```python
from build123d import *

# Parameters (mm, degrees)
SKETCH_1_R          = 18
SKETCH_1_R_2        = 1.6
SKETCH_1_R_3        = 2.6
SKETCH_1_R_4        = 1.35
EXTRUDE_1_DEPTH     = 3
CUT_EXTRUDE_1_REACH = 132.882
SKETCH_2_R          = 24


with BuildPart() as part:
    # 草图1 → 凸台-拉伸1 (new body)
    with BuildSketch(Plane(origin=(0, 0, 0), x_dir=(1, 0, 0), z_dir=(0, 1, 0))):
        with BuildLine():
            Line((100, -47.5), (-100, -47.5))
            ThreePointArc((-100, -47.5), (-121.921951267, 0), (-100, 47.5))
            Line((-100, 47.5), (100, 47.5))
            ThreePointArc((100, 47.5), (121.921951267, 0), (100, -47.5))
        make_face()
        with Locations(Location((77.5, 0, 0), (0, 0, 270))):
            Circle(SKETCH_1_R, mode=Mode.SUBTRACT)
        with Locations(Location((77.5, 37, 0), (0, 0, 270))):
            Circle(SKETCH_1_R_2, mode=Mode.SUBTRACT)
        with Locations(Location((103.662950904, 26.162950904, 0), (0, 0, 270))):
            Circle(SKETCH_1_R_2, mode=Mode.SUBTRACT)
        with Locations(Location((114.5, 0, 0), (0, 0, 270))):
            Circle(SKETCH_1_R_2, mode=Mode.SUBTRACT)
        with Locations(Location((103.662950904, -26.162950904, 0), (0, 0, 270))):
            Circle(SKETCH_1_R_2, mode=Mode.SUBTRACT)
        with Locations(Location((77.5, -37, 0), (0, 0, 270))):
            Circle(SKETCH_1_R_2, mode=Mode.SUBTRACT)
        with Locations(Location((51.337049096, -26.162950904, 0), (0, 0, 270))):
            Circle(SKETCH_1_R_2, mode=Mode.SUBTRACT)
        with Locations(Location((40.5, 0, 0), (0, 0, 270))):
            Circle(SKETCH_1_R_2, mode=Mode.SUBTRACT)
        with Locations(Location((51.337049096, 26.162950904, 0), (0, 0, 270))):
            Circle(SKETCH_1_R_2, mode=Mode.SUBTRACT)
        with Locations(Location((-51.337049096, 26.162950904, 0), (0, 0, 270))):
            Circle(SKETCH_1_R_2, mode=Mode.SUBTRACT)
        with Locations(Location((-40.5, 0, 0), (0, 0, 270))):
            Circle(SKETCH_1_R_2, mode=Mode.SUBTRACT)
        with Locations(Location((-51.337049096, -26.162950904, 0), (0, 0, 270))):
            Circle(SKETCH_1_R_2, mode=Mode.SUBTRACT)
        with Locations(Location((-77.5, -37, 0), (0, 0, 270))):
            Circle(SKETCH_1_R_2, mode=Mode.SUBTRACT)
        with Locations(Location((-103.662950904, -26.162950904, 0), (0, 0, 270))):
            Circle(SKETCH_1_R_2, mode=Mode.SUBTRACT)
        with Locations(Location((-114.5, 0, 0), (0, 0, 270))):
            Circle(SKETCH_1_R_2, mode=Mode.SUBTRACT)
        with Locations(Location((-103.662950904, 26.162950904, 0), (0, 0, 270))):
            Circle(SKETCH_1_R_2, mode=Mode.SUBTRACT)
        with Locations(Location((-77.5, 37, 0), (0, 0, 270))):
            Circle(SKETCH_1_R_2, mode=Mode.SUBTRACT)
        with Locations(Location((-77.5, 0, 0), (0, 0, 270))):
            Circle(SKETCH_1_R, mode=Mode.SUBTRACT)
        with Locations(Location((-10, -30.5, 0), (0, 0, 270))):
            Circle(SKETCH_1_R_3, mode=Mode.SUBTRACT)
        with Locations(Location((10, -30.5, 0), (0, 0, 270))):
            Circle(SKETCH_1_R_3, mode=Mode.SUBTRACT)
        with Locations(Location((-40, -30.5, 0), (0, 0, 270))):
            Circle(SKETCH_1_R_3, mode=Mode.SUBTRACT)
        with Locations(Location((40, -30.5, 0), (0, 0, 270))):
            Circle(SKETCH_1_R_3, mode=Mode.SUBTRACT)
        with Locations(Location((40, 30.5, 0), (0, 0, 270))):
            Circle(SKETCH_1_R_3, mode=Mode.SUBTRACT)
        with Locations(Location((10, 30.5, 0), (0, 0, 270))):
            Circle(SKETCH_1_R_3, mode=Mode.SUBTRACT)
        with Locations(Location((-10, 30.5, 0), (0, 0, 270))):
            Circle(SKETCH_1_R_3, mode=Mode.SUBTRACT)
        with Locations(Location((-40, 30.5, 0), (0, 0, 270))):
            Circle(SKETCH_1_R_3, mode=Mode.SUBTRACT)
        with Locations(Location((-30, -40.5, 0), (0, 0, 270))):
            Circle(SKETCH_1_R_2, mode=Mode.SUBTRACT)
        with Locations(Location((-40, -40.5, 0), (0, 0, 270))):
            Circle(SKETCH_1_R_2, mode=Mode.SUBTRACT)
        with Locations(Location((40, -40.5, 0), (0, 0, 270))):
            Circle(SKETCH_1_R_2, mode=Mode.SUBTRACT)
        with Locations(Location((30, -40.5, 0), (0, 0, 270))):
            Circle(SKETCH_1_R_2, mode=Mode.SUBTRACT)
        with Locations(Location((-40, 41, 0), (0, 0, 270))):
            Circle(SKETCH_1_R_2, mode=Mode.SUBTRACT)
        with Locations(Location((-30, 41, 0), (0, 0, 270))):
            Circle(SKETCH_1_R_2, mode=Mode.SUBTRACT)
        with Locations(Location((30, 41, 0), (0, 0, 270))):
            Circle(SKETCH_1_R_2, mode=Mode.SUBTRACT)
        with Locations(Location((40, 41, 0), (0, 0, 270))):
            Circle(SKETCH_1_R_2, mode=Mode.SUBTRACT)
        with Locations(Location((100, 37.5, 0), (0, 0, 270))):
            Circle(SKETCH_1_R_2, mode=Mode.SUBTRACT)
        with Locations(Location((100, -37.5, 0), (0, 0, 270))):
            Circle(SKETCH_1_R_2, mode=Mode.SUBTRACT)
        with Locations(Location((-100, -37.5, 0), (0, 0, 270))):
            Circle(SKETCH_1_R_2, mode=Mode.SUBTRACT)
        with Locations(Location((-100, 37.5, 0), (0, 0, 270))):
            Circle(SKETCH_1_R_2, mode=Mode.SUBTRACT)
        with Locations(Location((-30.5, 8, 0), (0, 0, 270))):
            Circle(SKETCH_1_R_4, mode=Mode.SUBTRACT)
        with BuildLine():
            Line((-36, 20), (-25, 20))
            ThreePointArc((-25, 20), (-23.585786438, 19.414213562), (-23, 18))
            Line((-23, 18), (-23, 12))
            ThreePointArc((-23, 12), (-23.585786438, 10.585786438), (-25, 10))
            Line((-25, 10), (-36, 10))
            ThreePointArc((-36, 10), (-37.414213562, 10.585786438), (-38, 12))
            Line((-38, 12), (-38, 18))
            ThreePointArc((-38, 18), (-37.414213562, 19.414213562), (-36, 20))
        make_face(mode=Mode.SUBTRACT)
    extrude(amount=EXTRUDE_1_DEPTH)

    # 草图2 → 切除-拉伸1 (cut, up to next)
    with BuildSketch(Plane(origin=(0, 3, 0), x_dir=(1, 0, 0), z_dir=(0, 1, 0)), mode=Mode.PRIVATE) as cut_extrude_1_sk1:
        with Locations(Location((77.5, 0, 0), (0, 0, 270))):
            Circle(SKETCH_2_R)
    cut_extrude_1_tool1 = extrude(cut_extrude_1_sk1.sketch, amount=-CUT_EXTRUDE_1_REACH, mode=Mode.PRIVATE) & part.part
    # 草图2 → 切除-拉伸1 (cut, up to next)
    with BuildSketch(Plane(origin=(0, 3, 0), x_dir=(1, 0, 0), z_dir=(0, 1, 0)), mode=Mode.PRIVATE) as cut_extrude_1_sk2:
        with Locations(Location((-77.5, 0, 0), (0, 0, 270))):
            Circle(SKETCH_2_R)
    cut_extrude_1_tool2 = extrude(cut_extrude_1_sk2.sketch, amount=-CUT_EXTRUDE_1_REACH, mode=Mode.PRIVATE) & part.part
    add(cut_extrude_1_tool1.solids().sort_by_distance((77.5, 3, 0))[0], mode=Mode.SUBTRACT)
    add(cut_extrude_1_tool2.solids().sort_by_distance((-77.5, 3, 0))[0], mode=Mode.SUBTRACT)


solid = part.part
```
Source: CAD feature listing. Evaluate the final solid. Frame: model axes, mm. Coordinates: 2 decimals unless noted, no trailing zeros. Write each loop counter-clockwise with the first axis right and the second up, starting at its lowest first coordinate (ties: lowest second). Pieces come first, ordered by that corner, then holes. Notation, with made-up numbers: (76.25, -28) - (81.25, -28) arc R14 cw to (81.25, -8) - close; hole circle Ø7 at (33.25, 5). An arc over 180 degrees is marked (long way). Answer as a JSON object with one key per item and string values.
Q1. Section query A-A, the plane z = -30.5. Output: boundary loops of the cut face in (x, y), plus the area to 3 significant figures.
Ans:
{"outline": "(-113.96, 0) - (-42.6, 0) - (-42.6, 3) - (-113.96, 3) - close; (-37.4, 0) - (-12.6, 0) - (-12.6, 3) - (-37.4, 3) - close; (-7.4, 0) - (7.4, 0) - (7.4, 3) - (-7.4, 3) - close; (12.6, 0) - (37.4, 0) - (37.4, 3) - (12.6, 3) - close; (42.6, 0) - (113.96, 0) - (113.96, 3) - (42.6, 3) - close", "area": "621 mm2"}
Q2. Section query D-D, the plane z = 31. Output: boundary loops of the cut face in (x, y), plus the area to 3 significant figures.
Ans:
{"outline": "(-113.68, 0) - (-42.55, 0) - (-42.55, 3) - (-113.68, 3) - close; (-37.45, 0) - (-12.55, 0) - (-12.55, 3) - (-37.45, 3) - close; (-7.45, 0) - (7.45, 0) - (7.45, 3) - (-7.45, 3) - close; (12.55, 0) - (37.45, 0) - (37.45, 3) - (12.55, 3) - close; (42.55, 0) - (113.68, 0) - (113.68, 3) - (42.55, 3) - close", "area": "621 mm2"}
Q3. Draft query along X for faces 1 (the cylindrical face through (-41.582, 1.479, -32.563)), 2 (the flat face through (2, 0, -1)), 3 (the cylindrical face through (8.418, 1.479, -32.563)), 4 (the cylindrical face through (-121.917, 1.479, 0.756)). Return one class per face: released by +X, released by -X, zero draft, split by the parting line, or undercut.
Ans:
{"face 1": "undercut", "face 2": "zero draft", "face 3": "undercut", "face 4": "released by -X"}
Q4. Section query B-B, the plane x = -73. Output: boundary loops of the cut face in (y, z), plus the area to 3 significant figures.
Ans:
{"outline": "(0, -47.5) - (3, -47.5) - (3, -23.57) - (0, -23.57) - close; (0, 23.57) - (3, 23.57) - (3, 47.5) - (0, 47.5) - close", "area": "144 mm2"}
Q5. Section query C-C, the plane z = 12. Output: boundary loops of the cut face in (x, y).
Ans:
{"outline": "(-120.76, 0) - (-98.28, 0) - (-98.28, 3) - (-120.76, 3) - close; (-56.72, 0) - (56.72, 0) - (56.72, 3) - (-56.72, 3) - close; (98.28, 0) - (120.76, 0) - (120.76, 3) - (98.28, 3) - close"}
Q6. Material intervals for line 1 (Z direction, x = -27, y = 0.8); line 2 (X direction, y = 0.25, z = 14.5); line 3 (X direction, y = 1.55, z = 20), sorted ascending. Write a range as [from, to].
Ans:
{"line 1": "z = [-47.5, -20], [-10, 47.5]", "line 2": "x = [-120.21, -96.62], [-58.38, 58.38], [96.62, 120.21]", "line 3": "x = [-118.63, -90.77], [-64.23, 64.23], [90.77, 118.63]"}
